Geometry: see drawing. Coordinates: mm, zero at the bounding-box minimum. A direction names the side the tool comes from. Give positions to 0.01 mm unless a question says otherwise; leave off trailing zeros. Write each loop counter-clockwise with the first axis right and the second up, starting at its lowest first coordinate (ties: lowest second). Pieces come first, ordered by that corner, then holes. Notation, with made-up numbers: (79.5, 8) - (116.5, 8) arc R25 ccw to (116.5, 20) - close; hole circle Ø3 at (0.25, 70.25). An arc over 180 degrees is marked (long way). Use a Markdown table: item, result. Add a question column.
1. Section query A-A, the plane z = 51.5. Return loops of the section in (x, y) (1 decimal), plus the area to 3 significant figures.
2. Section query B-B, the plane y = 88.9. Return loops of the section in (x, z) (1 decimal), plus the area to 3 significant figures.
3. Mould query, pull axis X, two halves, no side actions, for the marked faces 4, 5, 6 and 7. Classes: released by +X, released by -X, zero draft, split by the parting line, or undercut.
4. Section query D-D, the plane x = 44. Return loops of the section in (y, z).
5. Material intervals for probe 1 along X at (y, z) = (88, 20); probe 2 along Y at (x, z) = (18.5, 17); probe 3 along X at (y, z) = (42, 62) (1 decimal), sorted ascending.
6. Pin query (flat end, axial travel): pin 1 (1 mm diameter, centred on x = 10, z = 52.5, fed in from +Y); pin 2 (6 mm diameter, centred on x = 5.92, y = 88.9, fed in from -Z); pin 3 (4 mm diameter, centred on x = 37.5, z = 17.5, fed in from -Y). Return the tip coordinate at first contact, or that it passes through.
7. Set-up query: the marked faces 1, 2 and 3. Return all of +Z, -Z, +X, -X, +Y, -Y with unobstructed straight access to the full face (end or side cutting, diameter ignored); none if empty.
8. Section query C-C, the plane z = 5.5. Return loops of the section in (x, y) (1 decimal), plus the area to 3 significant figures.
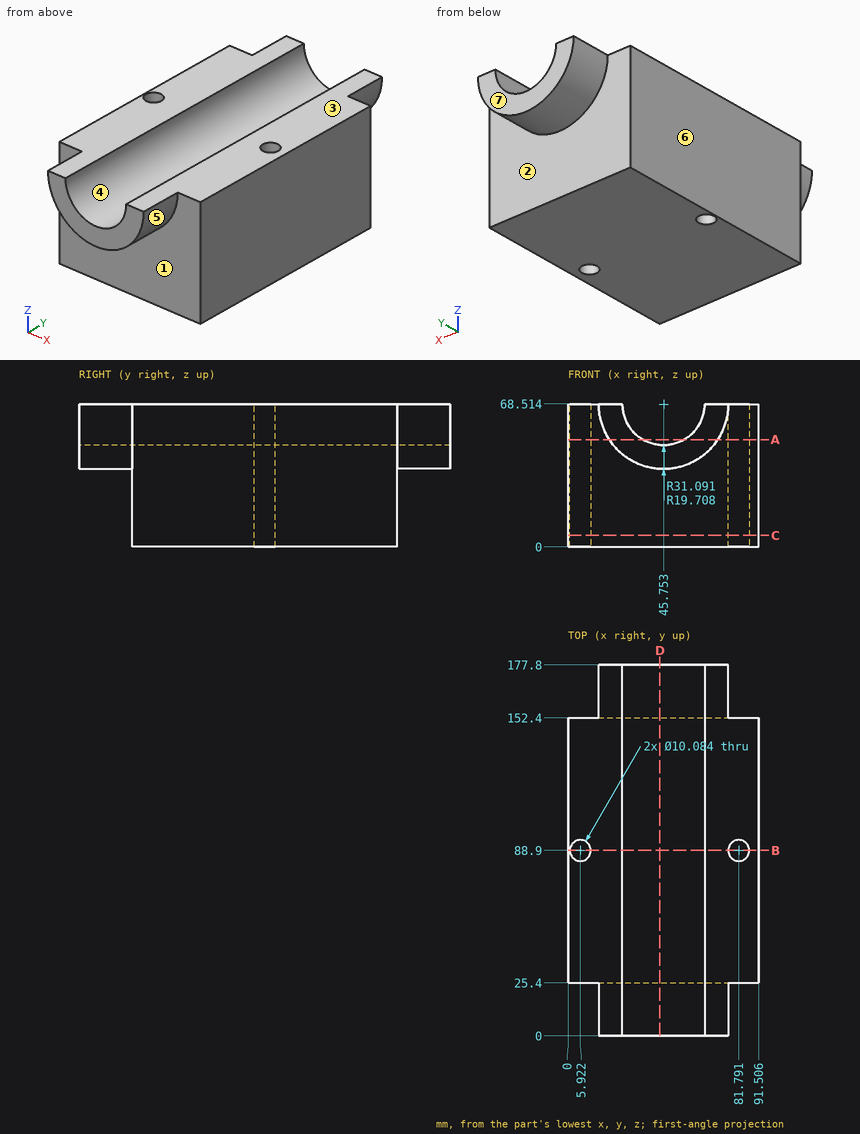
Result sheet:
| question | item | result |
|---|---|---|
| 1 | outline | (0, 25.4) - (19.7, 25.4) - (19.7, 0) - (35.8, 0) - (35.8, 177.8) - (19.7, 177.8) - (19.7, 152.4) - (0, 152.4) - close; (55.7, 0) - (71.8, 0) - (71.8, 25.4) - (91.5, 25.4) - (91.5, 152.4) - (71.8, 152.4) - (71.8, 177.8) - (55.7, 177.8) - close; hole circle Ø10.1 at (5.9, 88.9); hole circle Ø10.1 at (81.8, 88.9) |
| 1 | area | 10,600 mm² |
| 2 | outline | (0, 0) - (0.9, 0) - (0.9, 68.5) - (0, 68.5) - close; (11, 0) - (76.7, 0) - (76.7, 68.5) - (65.5, 68.5) arc R19.7 cw to (26, 68.5) - (11, 68.5) - close; (86.8, 0) - (91.5, 0) - (91.5, 68.5) - (86.8, 68.5) - close |
| 2 | area | 4,280 mm² |
| 3 | face 4 | undercut |
| 3 | face 5 | split by the parting line |
| 3 | face 6 | released by -X |
| 3 | face 7 | zero draft |
| 4 | outline | (0, 37.47) - (25.4, 37.47) - (25.4, 0) - (152.4, 0) - (152.4, 37.47) - (177.8, 37.47) - (177.8, 48.88) - (0, 48.88) - close |
| 5 | probe 1 | x = 0 to 0.96, 10.88 to 76.83, 86.75 to 91.51 |
| 5 | probe 2 | y = 25.4 to 152.4 |
| 5 | probe 3 | x = 0 to 27.2, 64.4 to 91.5 |
| 6 | pin 1 | stops at y = 152.4 |
| 6 | pin 2 | passes through |
| 6 | pin 3 | stops at y = 25.4 |
| 7 | face 1 | -Z, -Y |
| 7 | face 2 | -Z, +Y |
| 7 | face 3 | +Z, +X, -X, +Y, -Y |
| 8 | outline | (0, 25.4) - (91.5, 25.4) - (91.5, 152.4) - (0, 152.4) - close; hole circle Ø10.1 at (5.9, 88.9); hole circle Ø10.1 at (81.8, 88.9) |
| 8 | area | 11,500 mm² |
